from build123d import *

# Parameters (mm, degrees)
SKETCH1_W           = 27
SKETCH1_H           = 10
BOSS_EXTRUDE1_DEPTH = 9.8
CUT_EXTRUDE1_DEPTH  = 3.8
CUT_EXTRUDE2_DEPTH  = 3.8
HOLE1_D             = 3.4
HOLE1_DEPTH         = 9.8
HOLE2_D             = 3.4
HOLE2_DEPTH         = 9.8


with BuildPart() as part:
    # Sketch1 → Boss-Extrude1 (new body)
    with BuildSketch(Plane(origin=(0, 0, 0), x_dir=(-1, 0, 0), z_dir=(0, 0, -1))):
        with Locations((-8.5, 0)):
            Rectangle(SKETCH1_W, SKETCH1_H)
    extrude(amount=-BOSS_EXTRUDE1_DEPTH)

    # Sketch2 → Cut-Extrude1 (cut)
    with BuildSketch(Plane.XY.offset(9.8)):
        Polygon((-2.698076211, -1.557735027), (0, -3.115470054), (2.698076211, -1.557735027), (2.698076211, 1.557735027), (0, 3.115470054), (-2.698076211, 1.557735027), align=None)
    extrude(amount=-CUT_EXTRUDE1_DEPTH, mode=Mode.SUBTRACT)

    # Sketch3 → Cut-Extrude2 (cut)
    with BuildSketch(Plane.XY.offset(9.8)):
        Polygon((14.301923789, -1.557735027), (17, -3.115470054), (19.698076211, -1.557735027), (19.698076211, 1.557735027), (17, 3.115470054), (14.301923789, 1.557735027), align=None)
    extrude(amount=-CUT_EXTRUDE2_DEPTH, mode=Mode.SUBTRACT)

    # Hole1
    with Locations(Plane(origin=(0, 0, 0), x_dir=(-1, 0, 0), z_dir=(0, 0, -1))):
        with Locations((0, 0)):
            Hole(HOLE1_D / 2, depth=HOLE1_DEPTH)

    # Hole2
    with Locations(Plane(origin=(0, 0, 0), x_dir=(-1, 0, 0), z_dir=(0, 0, -1))):
        with Locations((-17, 0)):
            Hole(HOLE2_D / 2, depth=HOLE2_DEPTH)


solid = part.part
Can you work these out from the model? Positions are in its coordinate system, mm. A direction names the side the tool comes from. Coordinates: 2 decimals unless noted, no trailing zeros. Loops run counter-clockwise (first coordinate to the right, second up) from the corner with the lowest first, then second, coordinate; pieces in that order, holes last. Notation, with made-up numbers: M 73.5,60.5 L 77.5,60.5 A20 cw 77.5,66.5 Z; hole C -34,59.5 d11. An arc over 180 degrees is marked long. Return JSON: item names as keys, results as strings. Group by question number.
Item 1: Imagine slicing it at D-D (y = 2.5). Please give me the cut outline in (x, z).
Item 2: Thinking about a two-plate mould opening in X: for faces 1 (the flat face through (2, 0, 6)), 2 (the flat face through (22, 0, 5)), 3 (the flat face through (9, 5, 5)), which applies, released by +X, released by -X, zero draft, split by the parting line, or undercut?
Item 3: On a 3-axis mill with a long thin cutter (end or side, diameter ignored), from which of +Z, -Z, +X, -X, +Y, -Y can I reach the whole of each face in a straight line? I mean faces 4 (the cylindrical face through (18.57, -0.65, 3.04)), 5 (the flat face through (14.302, 0, 8)). Say none if no direction works.
Item 4: Imagine slicing it at C-C (x = 1.25). Please give me the cut outline in (y, z), and give its area (3 significant figures).
Item 5: I'm going to push a flat-ended pin straight in: pin 1 Ø1.6 at (x, y) = (16, -1.5) entering from +Z. Where does the tip first touch, or does it pass through?
Item 6: If I drill on L1, parallel to X at y = -1.5, z = 7.25; L2, parallel to Y at x = 17, z = 2.6; L3, parallel to X at y = 1, z = 0.5, over which ranges is the centre line in solid material (lowest first)? Write a range as from..to.
Item 7: Imagine slicing it at B-B (z = 7.25). Please give me the cut outline in (x, y).
Item 8: Imagine slicing it at A-A (y = 0). Please give me the cut outline in (x, z), and give its area (3 significant figures).
Verdict:
{
 "1": {"outline": "M -5,0 L 22,0 L 22,9.8 L 18.07,9.8 L 18.07,6 L 15.93,6 L 15.93,9.8 L 1.07,9.8 L 1.07,6 L -1.07,6 L -1.07,9.8 L -5,9.8 Z"},
 "2": {"face 1": "undercut", "face 2": "released by +X", "face 3": "zero draft"},
 "3": {"face 4": "+Z, -Z", "face 5": "+Z"},
 "4": {"outline": "M -5,0 L -1.15,0 L -1.15,6 L -2.39,6 L -2.39,9.8 L -5,9.8 Z; M 1.15,0 L 5,0 L 5,9.8 L 2.39,9.8 L 2.39,6 L 1.15,6 Z", "area": "66.0 mm^2"},
 "5": {"pin 1": "stops at z = 6"},
 "6": {"L1": "x = -5..-2.7, 2.7..14.3, 19.7..22", "L2": "y = -5..-1.7, 1.7..5", "L3": "x = -5..-1.37, 1.37..15.63, 18.37..22"},
 "7": {"outline": "M -5,-5 L 22,-5 L 22,5 L -5,5 Z; hole M -2.7,-1.56 L 0,-3.12 L 2.7,-1.56 L 2.7,1.56 L 0,3.12 L -2.7,1.56 Z; hole M 14.3,-1.56 L 17,-3.12 L 19.7,-1.56 L 19.7,1.56 L 17,3.12 L 14.3,1.56 Z"},
 "8": {"outline": "M -5,0 L -1.7,0 L -1.7,6 L -2.7,6 L -2.7,9.8 L -5,9.8 Z; M 1.7,0 L 15.3,0 L 15.3,6 L 14.3,6 L 14.3,9.8 L 2.7,9.8 L 2.7,6 L 1.7,6 Z; M 18.7,0 L 22,0 L 22,9.8 L 19.7,9.8 L 19.7,6 L 18.7,6 Z", "area": "183 mm^2"}
}
